```python
from build123d import *

# Parameters (mm, degrees)
CUT_EXTRUDE1_START = -1.5
CUT_EXTRUDE1_DEPTH = 1.5
SKETCH4_R          = 1.443375673
CUT_EXTRUDE2_DEPTH = 0.5
CUT_EXTRUDE2_TAPER = 45


with BuildPart() as part:
    # Sketch2 → Revolve1 (revolve)
    with BuildSketch(Plane(origin=(0, 0, 0), x_dir=(0, 0, -1), z_dir=(1, 0, 0))):
        Polygon((-9.35, 2.75), (-6.65, 2.75), (-6.5, 2.6), (-6.5, 1.5), (9, 1.5), (9.5, 1), (9.5, 0), (-9.5, 0), (-9.5, 2.6), align=None)
    revolve(axis=Axis((0, 0, -9.5), (0, 0, 1)))

    # Sketch3 → Cut-Extrude1 (cut)
    with BuildSketch(Plane.XY.offset(9.5).offset(CUT_EXTRUDE1_START)):
        Polygon((0, 1.443375673), (-1.25, 0.721687836), (-1.25, -0.721687836), (0, -1.443375673), (1.25, -0.721687836), (1.25, 0.721687836), align=None)
    extrude(amount=CUT_EXTRUDE1_DEPTH, mode=Mode.SUBTRACT)

    # Sketch4 → Cut-Extrude2 (cut)
    with BuildSketch(Plane.XY.offset(9.5)):
        Circle(SKETCH4_R)
    extrude(amount=-CUT_EXTRUDE2_DEPTH, taper=CUT_EXTRUDE2_TAPER, mode=Mode.SUBTRACT)


solid = part.part
```
Source: CAD feature listing. Evaluate the final solid. Frame: model axes, mm. A direction names the side the tool comes from. Give positions to 0.01 mm unless a question says otherwise; leave off trailing zeros. Order: outer loops, then holes, each group sorted by start corner. A loop starts at its lowest first (then second) coordinate and runs counter-clockwise, first axis right, second up.
(1) Section query B-B (z = 1.25). Return the cut outline in (x, y), plus the area to 3 significant figures.
(2) Access query for faces 4 (the face through (-0.07, -1.5, -1.36)), 5 (the face through (0, -2, 9.5)), 6 (the face through (-0.63, -1.08, 8.74)). Directions: +Z, -Z, +X, -X, +Y, -Y. A direction counts if a zero-diameter tool reaches every point of the face in a straight line with its end or side. Return the directions, or none.
(3) Contact query for flat-ended pins moving along their axis: P1, Ø2, axis at y = -1.5, z = 5, coming from the -X side; P2, Ø3, axis at x = 0.5, y = 0.5, coming from the +Z side; P3, Ø2, axis at x = -0.5, z = -3, coming from the +Y side. Output: stop coordinate, or through.
(4) Material intervals for line 1 along Z through (x, y) = (-1.65, -0.1); line 2 along Z through (x, y) = (0.5, 0.05); line 3 along Y through (x, z) = (-2.45, 7.25), sorted ascending.
(5) Pull-direction query (Y, two-part tool) for faces 1 (the face through (2.685, -0.596, 7.981)), 2 (the face through (-1.25, 0, 9)), 3 (the face through (0, 0, -9.5)); classes: +Y half, -Y half, draft (parallel to the pull), parting line (faces both ways), or undercut.
(6) Section query A-A (y = 0). Return the cut outline in (x, z).
Outcome:
1. outline: circle Ø3 at (0, 0)
1. area: 7.07 mm2
2. face 4: -Z
2. face 5: +Z, +X, -X, +Y, -Y
2. face 6: +Z
3. P1: stops at x = -1.41
3. P2: stops at z = 9.5
3. P3: stops at y = 1.5
4. line 1: z = 6.5 to 9.5
4. line 2: z = -9.5 to 8
4. line 3: y = -1.25 to 1.25
5. face 1: parting line
5. face 2: undercut
5. face 3: draft
6. outline: (-2.75, 6.65) - (-2.6, 6.5) - (-1.5, 6.5) - (-1.5, -9) - (-1, -9.5) - (1, -9.5) - (1.5, -9) - (1.5, 6.5) - (2.6, 6.5) - (2.75, 6.65) - (2.75, 9.35) - (2.6, 9.5) - (1.44, 9.5) - (1.25, 9.31) - (1.25, 8) - (-1.25, 8) - (-1.25, 9.31) - (-1.44, 9.5) - (-2.6, 9.5) - (-2.75, 9.35) - close
